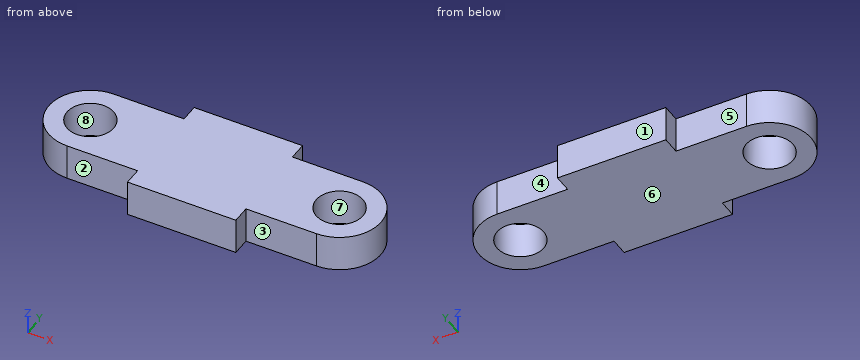
from build123d import *

# Parameters (mm, degrees)
SKETCH1_R           = 6.45
BOSS_EXTRUDE1_DEPTH = 10


with BuildPart() as part:
    # Sketch1 → Boss-Extrude1 (new body)
    with BuildSketch(Plane.XY):
        with BuildLine():
            Line((-39.617521433, 11.45), (-20.117521433, 11.45))
            Line((-20.117521433, 11.45), (-20.117521433, 16.45))
            Line((-20.117521433, 16.45), (9.882478567, 16.45))
            Line((9.882478567, 16.45), (9.882478567, 11.45))
            Line((9.882478567, 11.45), (29.382478567, 11.45))
            ThreePointArc((29.382478567, 11.45), (40.832478567, 0), (29.382478567, -11.45))
            Line((29.382478567, -11.45), (9.882478567, -11.45))
            Line((9.882478567, -11.45), (9.882478567, -16.45))
            Line((9.882478567, -16.45), (-20.117521433, -16.45))
            Line((-20.117521433, -16.45), (-20.117521433, -11.45))
            Line((-20.117521433, -11.45), (-39.617521433, -11.45))
            ThreePointArc((-39.617521433, -11.45), (-51.067521433, 0), (-39.617521433, 11.45))
        make_face()
        with Locations((-39.617521433, 0)):
            Circle(SKETCH1_R, mode=Mode.SUBTRACT)
        with Locations(Location((29.382478567, 0, 0), (0, 0, 180))):
            Circle(SKETCH1_R, mode=Mode.SUBTRACT)
    extrude(amount=-BOSS_EXTRUDE1_DEPTH)


solid = part.part
Here's how the part is built. I have some questions about the finished solid (model axes, mm). Face numbers are marked on the shaded views. A direction names the side the tool comes from. Coordinates: 2 decimals unless noted, no trailing zeros. Write each loop counter-clockwise with the first axis right and the second up, starting at its lowest first coordinate (ties: lowest second). Pieces come first, ordered by that corner, then holes.
Item 1: I want a section at B-B on y = 0. Write out the boundary of the cut face in (x, z).
Item 2: I want a section at C-C on y = 14.5. Write out the boundary of the cut face in (x, z), and give its area (3 significant figures).
Item 3: If we mould it in two halves opening along Y, with no side actions, what happens to the marked faces 5, 6, 7 and 8? For each: +Y half, -Y half, draft (parallel to the pull), parting line (faces both ways), or undercut.
Item 4: I want a section at A-A on z = -2.25. Write out the boundary of the cut face in (x, y).
Item 5: I want a section at D-D on x = 17. Write out the boundary of the cut face in (y, z).
Item 6: If I drill on line 1 (X direction, y = -1.5, z = -2); line 2 (X direction, y = -4, z = -8.25); line 3 (Y direction, x = 13.5, z = -9.5), over which ranges is the centre line in solid material (lowest first)?
Item 7: On a 3-axis mill with a long thin cutter (end or side, diameter ignored), from which of +Z, -Z, +X, -X, +Y, -Y can I reach the whole of each face in a straight line? I mean the marked faces 1, 2, 3 and 4. Say none if no direction works.
Item 8: Will these pins go through, and if not, where does the flat tip stop? pin 1 (1.5 mm diameter, centred on y = -14.5, z = -5.5, fed in from +X); pin 2 (1 mm diameter, centred on y = -5, z = -4.5, fed in from -X); pin 3 (5 mm diameter, centred on x = 21, z = -3, fed in from +Y); pin 4 (10.5 mm diameter, centred on x = 29.38, y = 0, fed in from +Z).
Findings below:
1. outline: (-51.07, -10) - (-46.07, -10) - (-46.07, 0) - (-51.07, 0) - close; (-33.17, -10) - (22.93, -10) - (22.93, 0) - (-33.17, 0) - close; (35.83, -10) - (40.83, -10) - (40.83, 0) - (35.83, 0) - close
2. outline: (-20.12, -10) - (9.88, -10) - (9.88, 0) - (-20.12, 0) - close
2. area: 300 mm2
3. face 5: +Y half
3. face 6: draft
3. face 7: undercut
3. face 8: undercut
4. outline: (-39.62, -11.45) - (-20.12, -11.45) - (-20.12, -16.45) - (9.88, -16.45) - (9.88, -11.45) - (29.38, -11.45) arc R11.45 ccw to (29.38, 11.45) - (9.88, 11.45) - (9.88, 16.45) - (-20.12, 16.45) - (-20.12, 11.45) - (-39.62, 11.45) arc R11.45 ccw to start; hole circle Ø12.9 at (-39.62, 0); hole circle Ø12.9 at (29.38, 0)
5. outline: (-11.45, -10) - (11.45, -10) - (11.45, 0) - (-11.45, 0) - close
6. line 1: x = -50.97 to -45.89, -33.34 to 23.11, 35.66 to 40.73
6. line 2: x = -50.35 to -44.68, -34.56 to 24.32, 34.44 to 40.11
6. line 3: y = -11.45 to 11.45
7. face 1: +Z, -Z, +X, -X, +Y
7. face 2: +Z, -Z, -X, -Y
7. face 3: +Z, -Z, +X, -Y
7. face 4: +Z, -Z, +X, +Y
8. pin 1: stops at x = 9.88
8. pin 2: stops at x = -50.15
8. pin 3: stops at y = 11.45
8. pin 4: passes through
